Part print with two shaded views. Sizes in mm from the minimum x, y, z corner. Round coordinates to 2 decimals unless told otherwise and drop trailing zeros. Loops run counter-clockwise (first coordinate to the right, second up) from the corner with the lowest first, then second, coordinate; pieces in that order, holes last. Notation, with made-up numbers: (71, 52.5) - (130, 52.5) arc R19 ccw to (130, 59.5) - close; hole circle Ø5 at (48, 35). An arc over 180 degrees is marked (long way). One line per question, with ' | ' between items.
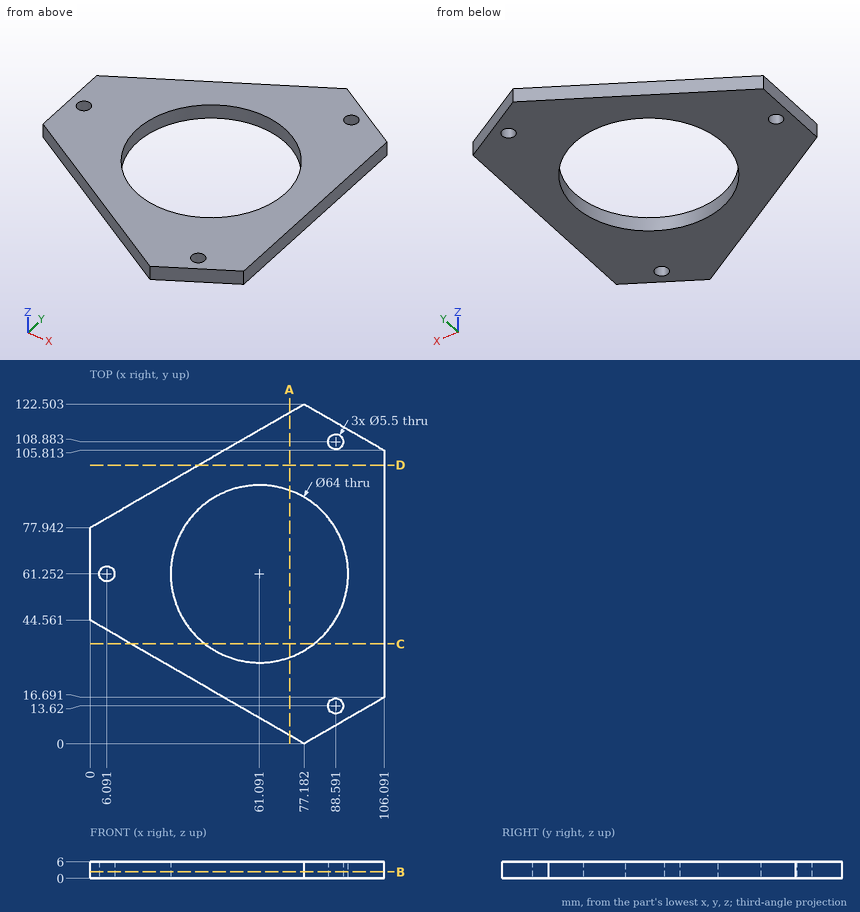
(1) Cut at A-A, the plane x = 72. Write the cut outline in (y, z) (1 decimal).
Results found:
outline: (3, 0) - (31.2, 0) - (31.2, 6) - (3, 6) - close; (91.3, 0) - (119.5, 0) - (119.5, 6) - (91.3, 6) - close
(2) Cut at D-D, the plane y = 100.5. Write the cut outline in (x, z).
Results found:
outline: (39.07, 0) - (106.09, 0) - (106.09, 6) - (39.07, 6) - close
(3) Probe L1, parallel to X at y = 60.5, z = 0.2 (1 decimal); L2, parallel to X at y = 89.5, z = 3.7 (1 decimal); L3, parallel to Y at x = 78, z = 2.8 (1 decimal). List the from-to ranges inside material, lowest first.
Results found:
L1: x = 0 to 3.4, 8.7 to 29.1, 93.1 to 106.1 | L2: x = 20 to 46.1, 76.1 to 106.1 | L3: y = 0.5 to 34.1, 88.4 to 122
(4) Cut at B-B, the plane z = 2.35. Write the cut outline in (x, y), then the cut area to 3 significant figures.
Results found:
outline: (0, 44.56) - (77.18, 0) - (106.09, 16.69) - (106.09, 105.81) - (77.18, 122.5) - (0, 77.94) - close; hole circle Ø5.5 at (6.09, 61.25); hole circle Ø64 at (61.09, 61.25); hole circle Ø5.5 at (88.59, 13.62); hole circle Ø5.5 at (88.59, 108.88) | area: 5,790 mm²
(5) Drop flat-ended pins along their axis: P1, Ø3, axis at x = 30.5, z = 3, coming from the -Y side (1 decimal); P2, Ø6.5, axis at x = 88.59, y = 13.62, coming from the +Z side; P3, Ø3.5, axis at x = 6.09, y = 61.25, coming from the -Z side; P4, Ø1, axis at x = 37, z = 4, coming from the +Y side. Give the stop position or say it passes through.
Results found:
P1: stops at y = 26.1 | P2: stops at z = 6 | P3: passes through | P4: stops at y = 99.59
(6) Cut at C-C, the plane y = 36. Write the cut outline in (x, z) (1 decimal), then the cut area to 3 significant figures.
Results found:
outline: (14.8, 0) - (41.4, 0) - (41.4, 6) - (14.8, 6) - close; (80.7, 0) - (106.1, 0) - (106.1, 6) - (80.7, 6) - close | area: 312 mm²
